Study the drawing (mm; zero at the part's minimum x, y, z) and answer. Give positions to 0.01 mm unless a question says otherwise; leave off trailing zeros. Write each loop counter-clockwise with the first axis right and the second up, starting at its lowest first coordinate (ties: lowest second). Pieces come first, ordered by that corner, then holes. Notation, with made-up numbers: M 46.25,55.5 L 75.25,55.5 A21 cw 75.25,87.5 Z; hole C 62.5,-35 d1. An arc over 180 degrees is marked long. Use a Markdown table: item, result. Add a question column.
Item 1: A cutting plane is placed at B-B on y = 7.75. Determine the outline of the cut face in (x, z), then the cut area to 3 significant figures.
Item 2: Consider probe 1 along Y at (x, z) = (3, 0.8) (1 decimal); probe 2 along X at (y, z) = (3.5, 1.6) (1 decimal); probe 3 along X at (y, z) = (2.5, 1.75) (1 decimal). Determine where each line is inside the solid, lowest interval first. Write a range as [from, to].
Item 3: Given P1, Ø1, axis at x = 1.5, y = 3, coming from the -Z side; P2, Ø3, axis at x = 4.1, y = 4.73, coming from the +Z side, each flat-ended and moving along its own axis, determine where each tip first touches the part or whether it passes through.
Item 4: A cutting plane is placed at A-A on z = 1.5. Determine the outline of the cut face in (x, y) (1 decimal), then the cut area to 3 significant figures.
Item 5: The mould has two halves that part along X. Classify the marked faces 1, 2, 3 and 4: pulls with the +X half, pulls with the -X half, needs draft (parallel to the pull), parting line crosses it, or undercut.
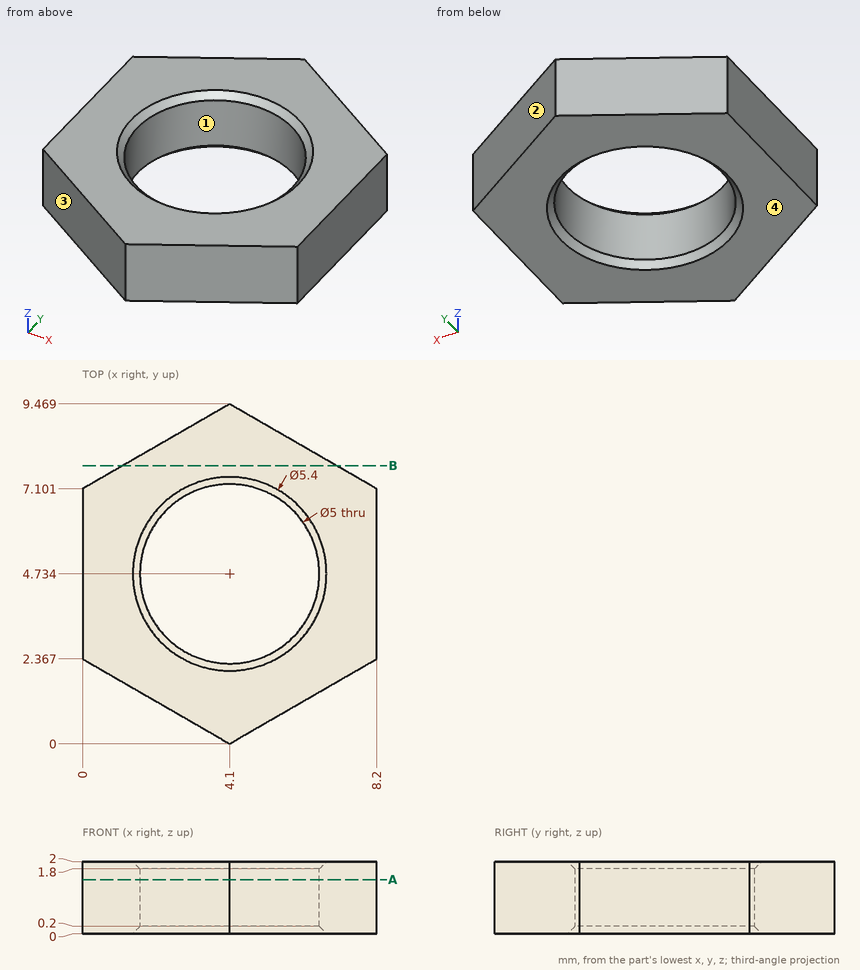
Filled in:
| question | item | result |
|---|---|---|
| 1 | outline | M 1.12,0 L 7.08,0 L 7.08,2 L 1.12,2 Z |
| 1 | area | 11.9 mm² |
| 2 | probe 1 | [0.6, 2.5], [7, 8.8] |
| 2 | probe 2 | [0, 1.9], [6.3, 8.2] |
| 2 | probe 3 | [0, 3], [5.2, 8.2] |
| 3 | P1 | z = 0 |
| 3 | P2 | through |
| 4 | outline | M 0,2.4 L 4.1,0 L 8.2,2.4 L 8.2,7.1 L 4.1,9.5 L 0,7.1 Z; hole C 4.1,4.7 d5 |
| 4 | area | 38.6 mm² |
| 5 | face 1 | undercut |
| 5 | face 2 | pulls with the +X half |
| 5 | face 3 | pulls with the -X half |
| 5 | face 4 | needs draft |
